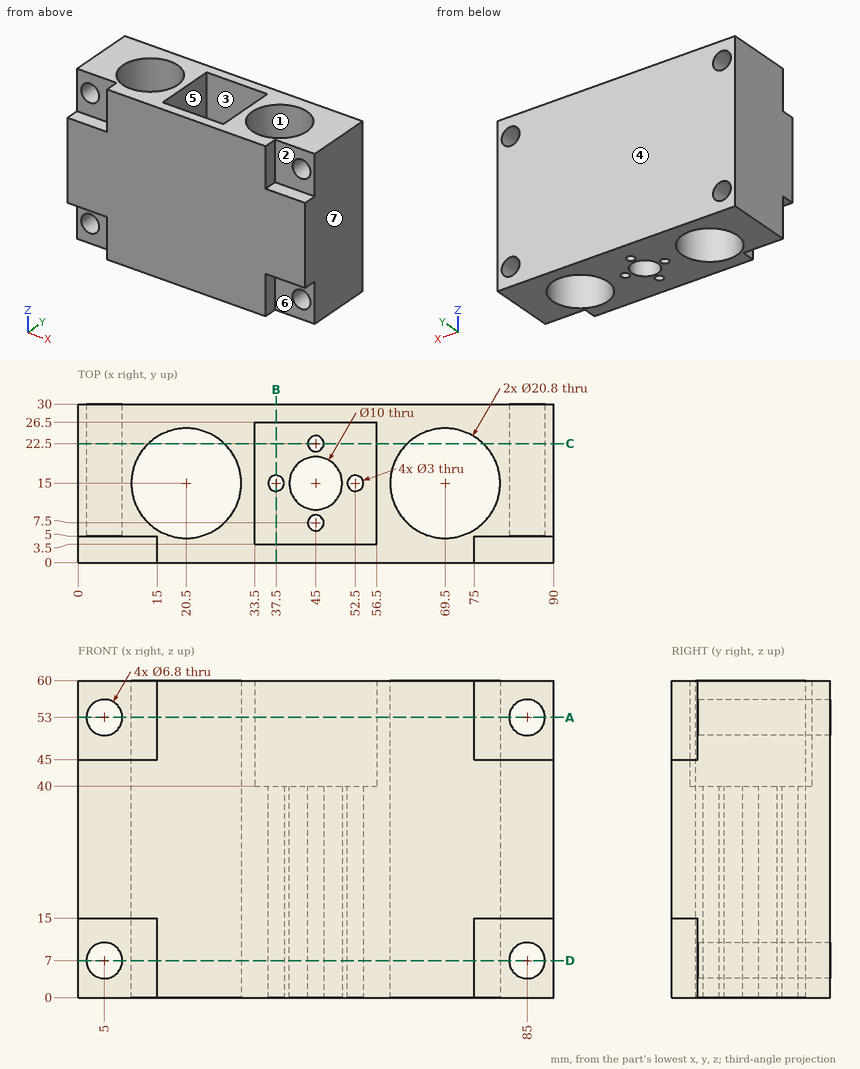
Can you work these out from the drawing? Everything is in mm from the part's minimum corner. A direction names the side the tool comes from. Round coordinates to 2 decimals unless told otherwise and drop trailing zeros. Order: outer loops, then holes, each group sorted by start corner. A loop starts at its lowest first (then second) coordinate and runs counter-clockwise, first axis right, second up. Notation, with made-up numbers: (-12.75, 62.5) - (30.25, 62.5) arc R26 cw to (30.25, 97.5) - close; hole circle Ø10 at (-39, 49.25). An arc over 180 degrees is marked (long way). Answer in a Markdown table with one row per item.
(1) Suppose I cut it at B-B, the plane x = 37.5. Please give me the cut outline in (y, z), plus the area to 3 significant figures.
From the geometry:
| item | result |
|---|---|
| outline | (0, 0) - (13.5, 0) - (13.5, 40) - (3.5, 40) - (3.5, 60) - (0, 60) - close; (16.5, 0) - (30, 0) - (30, 60) - (26.5, 60) - (26.5, 40) - (16.5, 40) - close |
| area | 1,220 mm2 |
(2) Suppose I cut it at A-A, the plane z = 53. Please give me the cut outline in (x, y), plus the area to 3 significant figures.
From the geometry:
| item | result |
|---|---|
| outline | (0, 5) - (1.6, 5) - (1.6, 30) - (0, 30) - close; (8.4, 5) - (15, 5) - (15, 0) - (75, 0) - (75, 5) - (81.6, 5) - (81.6, 30) - (8.4, 30) - close; (88.4, 5) - (90, 5) - (90, 30) - (88.4, 30) - close; hole circle Ø20.8 at (20.5, 15); hole (33.5, 3.5) - (56.5, 3.5) - (56.5, 26.5) - (33.5, 26.5) - close; hole circle Ø20.8 at (69.5, 15) |
| area | 1,000 mm2 |
(3) If we mould it in two halves opening along Y, with no side actions, what happens to the marked faces 4, 5, 6 and 7? For each: released by +Y, released by -Y, zero draft, split by the parting line, or undercut.
From the geometry:
| item | result |
|---|---|
| face 4 | released by +Y |
| face 5 | undercut |
| face 6 | released by -Y |
| face 7 | zero draft |
(4) Which directions (+Z, -Z, +X, -X, +Y, -Y) give clear straight access to the entire face, cutting with the end or side of a thin tool? Please do the marked faces 1, 2 and 3.
From the geometry:
| item | result |
|---|---|
| face 1 | +Z, -Z |
| face 2 | +Z, +X, -Y |
| face 3 | +Z |
(5) For P1, Ø1.5, axis at y = 2, z = 7.5, coming from the +X side; P2, Ø4, axis at x = 9.5, y = 2, coming from the +Z side; P3, Ø9, axis at x = 5, z = 7, coming from the -Y side; P4, Ø1.8, axis at x = 45, y = 22.5, coming from the -Z side, each with a flat end and sliding along its axis, tell me the tip position at first contact or that it passes through.
From the geometry:
| item | result |
|---|---|
| P1 | stops at x = 75 |
| P2 | stops at z = 45 |
| P3 | stops at y = 5 |
| P4 | passes through |
(6) Please list where these lines run through material, in increasing order: L1, parallel to Y at x = 45, z = 26.5; L2, parallel to Z at x = 5, y = 14.5; L3, parallel to Y at x = 37.5, z = 20. Write a range as from..to.
From the geometry:
| item | result |
|---|---|
| L1 | y = 0..6, 9..10, 20..21, 24..30 |
| L2 | z = 0..3.6, 10.4..49.6, 56.4..60 |
| L3 | y = 0..13.5, 16.5..30 |
(7) Suppose I cut it at D-D, the plane z = 7. Count the separate pieces of the cut face and the enclosed holes in it, plus the area to 3 significant figures.
From the geometry:
| item | result |
|---|---|
| separate pieces | 3 |
| enclosed holes | 7 |
| area | 1,420 mm2 |
(8) Suppose I cut it at C-C, the plane y = 22.5. Please give me the cut outline in (x, z).
From the geometry:
| item | result |
|---|---|
| outline | (0, 0) - (13.3, 0) - (13.3, 60) - (0, 60) - close; (27.7, 0) - (43.5, 0) - (43.5, 40) - (33.5, 40) - (33.5, 60) - (27.7, 60) - close; (46.5, 0) - (62.3, 0) - (62.3, 60) - (56.5, 60) - (56.5, 40) - (46.5, 40) - close; (76.7, 0) - (90, 0) - (90, 60) - (76.7, 60) - close; hole circle Ø6.8 at (5, 7); hole circle Ø6.8 at (5, 53); hole circle Ø6.8 at (85, 7); hole circle Ø6.8 at (85, 53) |
